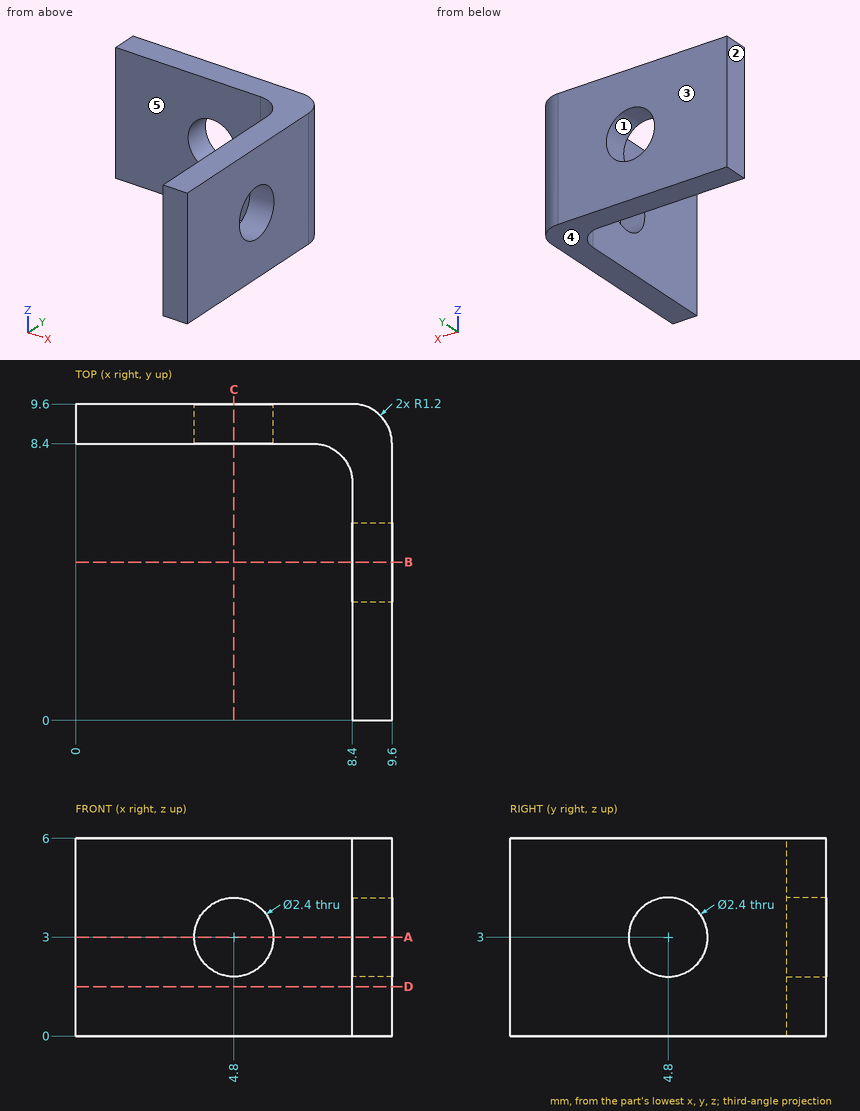
The figure shows three views and two pictorial views of one solid part (mm, origin at its lowest corner). Answer the questions. A direction names the side the tool comes from. Coordinates: 2 decimals unless noted, no trailing zeros. Loops run counter-clockwise (first coordinate to the right, second up) from the corner with the lowest first, then second, coordinate; pieces in that order, holes last.
(1) Consider line 1 along X through (y, z) = (0.75, 1.4); line 2 along Y through (x, z) = (9, 3). Determine where each line is inside the solid, lowest interval first.
Solution:
line 1: x = 8.4 to 9.6
line 2: y = 0 to 3.6, 6 to 9.44
(2) The part is cut by section B-B (y = 4.8). Determine the outline of the cut face in (x, z).
Solution:
outline: (8.4, 0) - (9.6, 0) - (9.6, 1.8) - (8.4, 1.8) - close; (8.4, 4.2) - (9.6, 4.2) - (9.6, 6) - (8.4, 6) - close
(3) The part is cut by section A-A (z = 3). Determine the outline of the cut face in (x, y), and give its area (3 significant figures).
Solution:
outline: (0, 8.4) - (3.6, 8.4) - (3.6, 9.6) - (0, 9.6) - close; (6, 8.4) - (7.2, 8.4) arc R1.2 cw to (8.4, 7.2) - (8.4, 6) - (9.6, 6) - (9.6, 8.4) arc R1.2 ccw to (8.4, 9.6) - (6, 9.6) - close; (8.4, 0) - (9.6, 0) - (9.6, 3.6) - (8.4, 3.6) - close
area: 15.8 mm2
(4) The mould has two halves that part along X. Classify the marked faces 1, 2 and 3: released by +X, released by -X, zero draft, split by the parting line, or undercut.
Solution:
face 1: undercut
face 2: released by -X
face 3: zero draft
(5) The part is cut by section D-D (z = 1.5). Determine the outline of the cut face in (x, y).
Solution:
outline: (0, 8.4) - (7.2, 8.4) arc R1.2 cw to (8.4, 7.2) - (8.4, 0) - (9.6, 0) - (9.6, 8.4) arc R1.2 ccw to (8.4, 9.6) - (0, 9.6) - close
(6) A tool of negligible diameter and unlimited length cuts with its end or side. For the marked faces 4 and 5, from which of +Z, -Z, +X, -X, +Y, -Y can it reach the whole face along a straight path? Write none if from no direction.
Solution:
face 4: -Z, +X, -X, +Y, -Y
face 5: +Z, -Z, -X, -Y
(7) A flat-ended cylindrical pin translates along its axis: pin 1 Ø3 at (y, z) = (4.8, 3) entering from +X. Find the tip coordinate at first contact, or state that the pin passes through.
Solution:
pin 1: stops at x = 9.6
